```python
from build123d import *

# Parameters (mm, degrees)
SKETCH1_R           = 37.5
SKETCH1_R_2         = 2.25
BOSS_EXTRUDE1_DEPTH = 10
SKETCH4_R           = 17.5
CUT_EXTRUDE3_DEPTH  = 6
CUT_EXTRUDE1_DEPTH  = 6
CUT_EXTRUDE2_DEPTH  = 10
FILLET1_R           = 3


with BuildPart() as part:
    # Sketch1 → Boss-Extrude1 (new body)
    with BuildSketch(Plane(origin=(0, 0, 0), x_dir=(1, 0, 0), z_dir=(0, 1, 0))):
        Circle(SKETCH1_R)
        with Locations((0, 27.5)):
            Circle(SKETCH1_R_2, mode=Mode.SUBTRACT)
        with Locations((23.815698604, 13.75)):
            Circle(SKETCH1_R_2, mode=Mode.SUBTRACT)
        with Locations((23.815698604, -13.75)):
            Circle(SKETCH1_R_2, mode=Mode.SUBTRACT)
        with Locations((0, -27.5)):
            Circle(SKETCH1_R_2, mode=Mode.SUBTRACT)
        with Locations((-23.815698604, -13.75)):
            Circle(SKETCH1_R_2, mode=Mode.SUBTRACT)
        with Locations((-23.815698604, 13.75)):
            Circle(SKETCH1_R_2, mode=Mode.SUBTRACT)
    extrude(amount=BOSS_EXTRUDE1_DEPTH)

    # Sketch4 → Cut-Extrude3 (cut)
    with BuildSketch(Plane(origin=(0, 10, 0), x_dir=(1, 0, 0), z_dir=(0, 1, 0))):
        Circle(SKETCH4_R)
    extrude(amount=-CUT_EXTRUDE3_DEPTH, mode=Mode.SUBTRACT)

    # Sketch2 → Cut-Extrude1 (cut)
    with BuildSketch(Plane(origin=(0, 10, 0), x_dir=(1, 0, 0), z_dir=(0, 1, 0))):
        with BuildLine():
            Line((-37.468790286, 1.529625603), (-17.383968992, -2.011870294))
            ThreePointArc((-17.383968992, -2.011870294), (-17.234135678, 3.038843109), (-15.647487215, 7.836207236))
            Line((-15.647487215, 7.836207236), (-35.73230851, 11.377703133))
            ThreePointArc((-35.73230851, 11.377703133), (-36.930290738, 6.511806663), (-37.468790286, 1.529625603))
        make_face()
    extrude(amount=-CUT_EXTRUDE1_DEPTH, mode=Mode.SUBTRACT)

    # Sketch3 → Cut-Extrude2 (cut)
    with BuildSketch(Plane.XZ):
        with BuildLine():
            Line((-37.5, 0), (-18.75, 32.475952642))
            ThreePointArc((-18.75, 32.475952642), (-32.475952642, 18.75), (-37.5, 0))
        make_face()
    extrude(amount=-CUT_EXTRUDE2_DEPTH, mode=Mode.SUBTRACT)

    # Fillet1
    fillet1_edges = [part.edges().sort_by_distance(p)[0] for p in [
        (17.234135678, 4, 3.038843109),
        (-27.426379639, 4, 0.241122346),
        (-15.647487215, 7, -7.836207236),
        (-25.689897863, 4, -9.606955184),
        (-17.383968992, 7, 2.011870294),
        (-18.75, 5, 32.475952642),
        (-37.5, 5, 0),
    ]]
    fillet(fillet1_edges, radius=FILLET1_R)


solid = part.part
```
Geometry: final body of the model. Coordinates: model frame, mm. A direction names the side the tool comes from. Round coordinates to 2 decimals unless told otherwise and drop trailing zeros. Loops run counter-clockwise (first coordinate to the right, second up) from the corner with the lowest first, then second, coordinate; pieces in that order, holes last. Notation, with made-up numbers: (1, 80) -> (27, 80) arc R14 cw to (27, 98) -> close; hole circle Ø9 at (-21.75, 78.5). An arc over 180 degrees is marked (long way). Use one line per item in the form item = value. Start each with the question number.
1) Section C-C on z = -27.5. Output: boundary loops of the cut face in (x, y), then the cut area to 3 significant figures.
2) Draft query along X for faces 4 (the cylindrical face through (-21.67, 4.93, 13.07)), 5 (the flat face through (-1, 0, -1)), 6 (the flat face through (-26.6, 8.521, -9.767)). Return one class per face: released by +X, released by -X, zero draft, split by the parting line, or undercut.
3) Section A-A on x = 0. Output: boundary loops of the cut face in (y, z), then the cut area to 3 significant figures.
4) Access query for faces 1 (the cylindrical face through (-27.149, 4.855, -8.948)), 2 (the cylindrical face through (-0.488, 4.93, 29.696)), 3 (the flat face through (-6, 4, 0)). Directions: +Z, -Z, +X, -X, +Y, -Y. A direction counts if a zero-diameter tool reaches every point of the face in a straight line with its end or side. Return the directions, or none.
5) Section B-B on y = 1.25. Output: boundary loops of the cut face in (x, z), then the cut area to 3 significant figures.
6) Section D-D on x = 23. Output: boundary loops of the cut face in (y, z), then the cut area to 3 significant figures.
7) First-contact query: P1, Ø3, axis at x = 24, y = 1.5, coming from the +Z side; P2, Ø5, axis at x = 11.5, y = 2, coming from the +Z side; P3, Ø8.5, axis at x = -18.5, z = -3, coming from the +Y side. Flat tips, straight axial feed; report the tip coordinate or a pass-through.
8) Line query: L1, parallel to Z at x = 0, y = 8.9; L2, parallel to Z at x = 1, y = 2.25; L3, parallel to Y at x = 12.5, z = -7.5. Output: solid intervals per line, ascending.
Response:
q1.outline = (-25.5, 0) -> (-2.25, 0) -> (-2.25, 10) -> (-25.5, 10) -> close; (2.25, 0) -> (25.5, 0) -> (25.5, 10) -> (2.25, 10) -> close
q1.area = 465 mm^2
q2.face_4 = undercut
q2.face_5 = zero draft
q2.face_6 = released by -X
q3.outline = (0, -37.5) -> (10, -37.5) -> (10, -29.75) -> (0, -29.75) -> close; (0, -25.25) -> (10, -25.25) -> (10, -17.5) -> (7, -17.5) arc R3 cw to (4, -14.5) -> (4, 14.5) arc R3 cw to (7, 17.5) -> (10, 17.5) -> (10, 25.25) -> (0, 25.25) -> close; (0, 29.75) -> (10, 29.75) -> (10, 37.5) -> (0, 37.5) -> close
q3.area = 454 mm^2
q4.face_1 = -X, +Y
q4.face_2 = +Y, -Y
q4.face_3 = +Y
q5.outline = (-37.49, -0.86) arc R37.5 ccw (long way) to (-18, 32.9) arc R3 ccw to (-19.16, 31.76) -> (-37.09, 0.71) arc R3 ccw to start; hole circle Ø4.5 at (-23.82, -13.75); hole circle Ø4.5 at (-23.82, 13.75); hole circle Ø4.5 at (0, -27.5); hole circle Ø4.5 at (0, 27.5); hole circle Ø4.5 at (23.82, -13.75); hole circle Ø4.5 at (23.82, 13.75)
q5.area = 4,190 mm^2
q6.outline = (0, -29.62) -> (10, -29.62) -> (10, -15.85) -> (0, -15.85) -> close; (0, -11.65) -> (10, -11.65) -> (10, 11.65) -> (0, 11.65) -> close; (0, 15.85) -> (10, 15.85) -> (10, 29.62) -> (0, 29.62) -> close
q6.area = 508 mm^2
q7.P1 = 30
q7.P2 = 36.4
q7.P3 = 5.35
q8.L1 = -37.5 to -29.75, -25.25 to -17.5, 17.5 to 25.25, 29.75 to 37.5
q8.L2 = -37.49 to -29.52, -25.48 to 25.48, 29.52 to 37.49
q8.L3 = 0 to 4
